Geometry: see drawing. Coordinates: mm, zero at the bounding-box minimum. A direction names the side the tool comes from. Round coordinates to 2 decimals unless told otherwise and drop trailing zeros. Loops run counter-clockwise (first coordinate to the right, second up) from the corner with the lowest first, then second, coordinate; pieces in that order, holes last. Notation, with made-up numbers: (57.5, 23) - (80.5, 23) arc R24 ccw to (80.5, 58) - close; hole circle Ø10 at (71, 56.25). An arc over 180 degrees is marked (long way). Write item = value, one per line. Start each with the question number.
Item 1: Section B-B (y = 14.75). Return loops of the section in (x, z).
Item 2: Access query for the marked faces 1, 2 and 3. Directions: +Z, -Z, +X, -X, +Y, -Y. A direction counts if a zero-diameter tool reaches every point of the face in a straight line with its end or side. Return the directions, or none.
Item 3: Line query: line 1 (X direction, y = 7.5, z = 6.25); line 2 (Z direction, x = 1.25, y = 1.5); line 3 (Z direction, x = 3.75, y = 20.25) (1 decimal). Output: solid intervals per line, ascending. Write a range as from..to.
Item 4: Section A-A (x = 6). Return loops of the section in (y, z), plus the area to 3 significant figures.
Item 5: Section D-D (x = 21). Return loops of the section in (y, z).
Item 6: Section C-C (z = 7.5). Return loops of the section in (x, y).
Item 7: Draft query along Z for the marked faces 4, 5 and 6. Return one class per face: pulls with the +Z half, pulls with the -Z half, needs draft (parallel to the pull), parting line crosses it, or undercut.
Item 8: First-contact query: pin 1 (2 mm diameter, centred on y = 6.5, z = 7.5, fed in from +X); pin 2 (3 mm diameter, centred on y = 21.5, z = 5.5, fed in from +X); pin 3 (1 mm diameter, centred on y = 13.5, z = 2.5, fed in from -X). Flat tips, straight axial feed; report the tip coordinate or a pass-through.
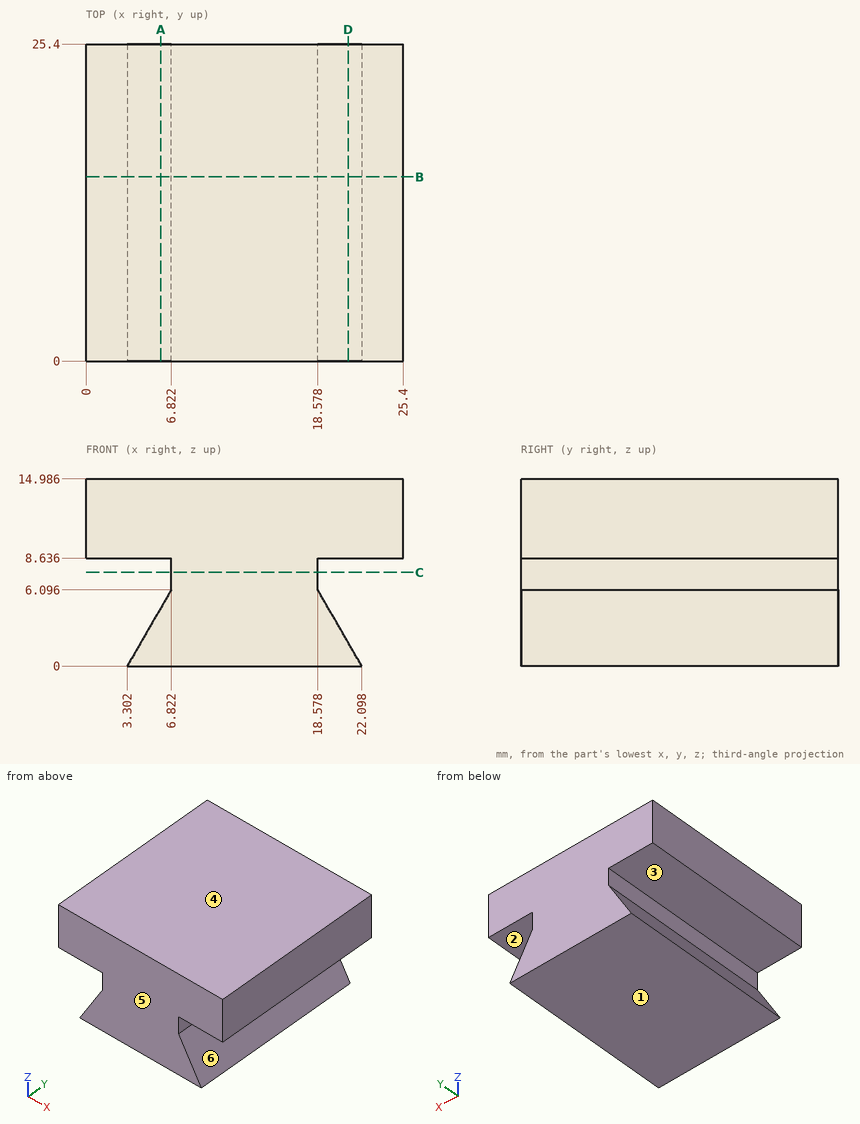
Taken from the geometry:
q1.outline = (0, 8.64) - (6.82, 8.64) - (6.82, 6.1) - (3.3, 0) - (22.1, 0) - (18.58, 6.1) - (18.58, 8.64) - (25.4, 8.64) - (25.4, 14.99) - (0, 14.99) - close
q2.face_1 = -Z, +X, -X, +Y, -Y
q2.face_2 = +X, +Y, -Y
q2.face_3 = -X, +Y, -Y
q3.line_1 = 6.82..18.58
q3.line_2 = 8.64..14.99
q3.line_3 = 0..0.8, 8.6..15
q4.outline = (0, 0) - (25.4, 0) - (25.4, 4.67) - (0, 4.67) - close; (0, 8.64) - (25.4, 8.64) - (25.4, 14.99) - (0, 14.99) - close
q4.area = 280 mm^2
q5.outline = (0, 0) - (25.4, 0) - (25.4, 1.9) - (0, 1.9) - close; (0, 8.64) - (25.4, 8.64) - (25.4, 14.99) - (0, 14.99) - close
q6.outline = (6.82, 0) - (18.58, 0) - (18.58, 25.4) - (6.82, 25.4) - close
q7.face_4 = pulls with the +Z half
q7.face_5 = needs draft
q7.face_6 = undercut
q8.pin_1 = 18.58
q8.pin_2 = 19.79
q8.pin_3 = 4.46
